Check sheet for the modelled part. Datum: model origin and axes. Units: mm. Face numbers are marked on the shaded views. A direction names the side the tool comes from. Give positions to 0.01 mm unless a question says otherwise; leave off trailing zeros. Write each loop counter-clockwise with the first axis right and the second up, starting at its lowest first coordinate (ties: lowest second). Pieces come first, ordered by that corner, then holes. Notation, with made-up numbers: M 31,-30 L 86,-30 A12 ccw 86,-20 Z; hole C 41,23 d10. An arc over 180 degrees is marked long. Write item = value, one per line. Start each with the question number.
1) Cross-section at C-C, the plane z = 9.5. Record the cut outline in (x, y), plus the area to 3 significant figures.
2) Access from +Z, -Z, +X, -X, +Y, -Y to the whole of each face (thin tool, end or side, straight path). Record for the marked faces 5 and 6.
3) Scan lines: line 1 along Y through (x, z) = (0, 7.4); line 2 along Y through (x, z) = (0, 2.9); line 3 along Z through (x, y) = (12, 10). Record each from-to range of solid material in increasing order. Write a range as [from, to].
4) Mould release check, pull along Y, two halves, no side actions. Record for the marked faces 1, 2, 3 and 4: released by +Y, released by -Y, zero draft, split by the parting line, or undercut.
5) Go/stop test with flat-tipped pins: pin 1 (17.5 mm diameter, centred on x = -0.5, y = 0.5, fed in from -Z); pin 2 (1.5 mm diameter, centred on x = -10, y = 7.5, fed in from -Z); pin 3 (8 mm diameter, centred on x = -4.5, y = -3, fed in from -Z); pin 4 (2 mm diameter, centred on x = 4.5, z = 2.5, fed in from +Y). Record where each tip stops, or that it passes through.
6) Cross-section at A-A, the plane x = 0. Record the cut outline in (y, z), plus the area to 3 significant figures.
```python
from build123d import *

# Parameters (mm, degrees)
F3_D     = 4.2
F3_DEPTH = 10
F3_TIP   = 1.2618073
F4_SIZE  = 1
F5_SIZE  = 2


with BuildPart() as f1:
    # F0 (on Front) → F1 (revolve)
    with BuildSketch(Plane.XZ):
        Polygon((17, 10.5), (0, 10.5), (0, 5.5), (8, 5.5), (8, 0), (13.7, 0), (13.7, 3), (12, 3), (12, 5.5), (13.7, 5.5), (13.7, 8.5), (17, 8.5), align=None)
    revolve(axis=Axis((0, 0, 19.6601920579), (0, 0, 1)))

    # F3
    with Locations(Plane.XY.offset(10.5)):
        with Locations((0, 0)):
            Hole(F3_D / 2, depth=F3_DEPTH)
            with Locations((0, 0, -(F3_DEPTH + F3_TIP / 2))):  # 118° drill point
                Cone(0, F3_D / 2, F3_TIP, mode=Mode.SUBTRACT)

    # F4
    f4_edges = [f1.edges().sort_by_distance(p)[0] for p in [
        (-13.7, 0, 0),
    ]]
    chamfer(f4_edges, length=F4_SIZE)

    # F5
    f5_edges = [f1.edges().sort_by_distance(p)[0] for p in [
        (-8, 0, 0),
    ]]
    chamfer(f5_edges, length=F5_SIZE)


solid = f1.part
```
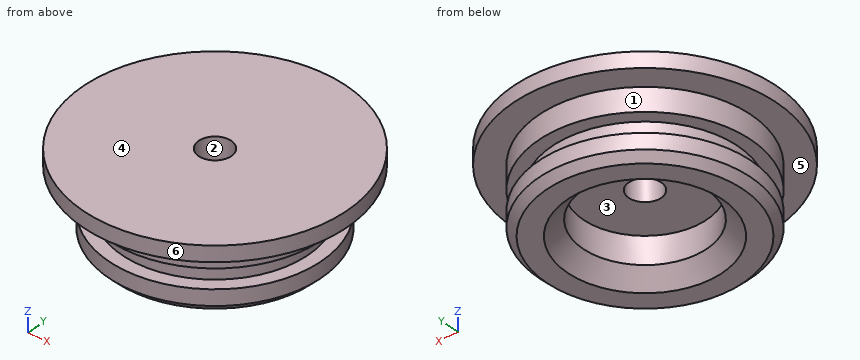
Reply:
q1.outline = C 0,0 d34; hole C 0,0 d4.2
q1.area = 894 mm2
q2.face_5 = -Z
q2.face_6 = +Z, -Z
q3.line_1 = [-13.7, -2.1], [2.1, 13.7]
q3.line_2 = [-13.7, -8], [8, 13.7]
q3.line_3 = [8.5, 10.5]
q4.face_1 = split by the parting line
q4.face_2 = undercut
q4.face_3 = undercut
q4.face_4 = zero draft
q5.pin_1 = 0.54
q5.pin_2 = 0
q5.pin_3 = 0.59
q5.pin_4 = 13.25
q6.outline = M -17,8.5 L -13.7,8.5 L -13.7,5.5 L -12,5.5 L -12,3 L -13.7,3 L -13.7,1 L -12.7,0 L -10,0 L -8,2 L -8,5.5 L -2.1,5.5 L -2.1,10.5 L -17,10.5 Z; M 2.1,5.5 L 8,5.5 L 8,2 L 10,0 L 12.7,0 L 13.7,1 L 13.7,3 L 12,3 L 12,5.5 L 13.7,5.5 L 13.7,8.5 L 17,8.5 L 17,10.5 L 2.1,10.5 Z
q6.area = 178 mm2
